```python
from build123d import *

# Parameters (mm, degrees)
SKETCH7_W           = 100
SKETCH7_H           = 14.5
BOSS_EXTRUDE1_DEPTH = 16.5
SKETCH8_R           = 5
CUT_EXTRUDE2_DEPTH  = 13
SKETCH10_R          = 13
CUT_EXTRUDE3_DEPTH  = 2
FILLET1_R           = 3
FILLET3_R           = 3
FILLET4_R           = 3
FILLET5_R           = 3


with BuildPart() as part:
    # Sketch7 → Boss-Extrude1 (new body)
    with BuildSketch(Plane(origin=(0, 0, 0), x_dir=(0, 1, 0), z_dir=(0, 0, 1))):
        Rectangle(SKETCH7_W, SKETCH7_H)
    extrude(amount=BOSS_EXTRUDE1_DEPTH)

    # Sketch8 → Cut-Extrude2 (cut)
    with BuildSketch(Plane(origin=(0, 0, 16.5), x_dir=(0, -1, 0), z_dir=(0, 0, 1))):
        with Locations(Location((0, 0, 0), (0, 0, 90))):
            Circle(SKETCH8_R)
    extrude(amount=-CUT_EXTRUDE2_DEPTH, mode=Mode.SUBTRACT)

    # Sketch10 → Cut-Extrude3 (cut)
    with BuildSketch(Plane.XY.offset(16.5)):
        with Locations((0, -31.55)):
            Circle(SKETCH10_R)
    cut_extrude3 = extrude(amount=-CUT_EXTRUDE3_DEPTH, mode=Mode.SUBTRACT)

    # Mirror1: Cut-Extrude3 across plane
    add(cut_extrude3.mirror(Plane.ZX), mode=Mode.SUBTRACT)

    # Fillet1
    fillet1_edges = [part.edges().sort_by_distance(p)[0] for p in [
        (-7.25, 0, 0),
    ]]
    fillet(fillet1_edges, radius=FILLET1_R)

    # Fillet3
    fillet3_edges = [part.edges().sort_by_distance(p)[0] for p in [
        (7.25, 0, 0),
    ]]
    fillet(fillet3_edges, radius=FILLET3_R)

    # Fillet4
    fillet4_edges = [part.edges().sort_by_distance(p)[0] for p in [
        (0, 50, 16.5),
    ]]
    fillet(fillet4_edges, radius=FILLET4_R)

    # Fillet5
    fillet5_edges = [part.edges().sort_by_distance(p)[0] for p in [
        (0, -50, 16.5),
    ]]
    fillet(fillet5_edges, radius=FILLET5_R)


solid = part.part
```
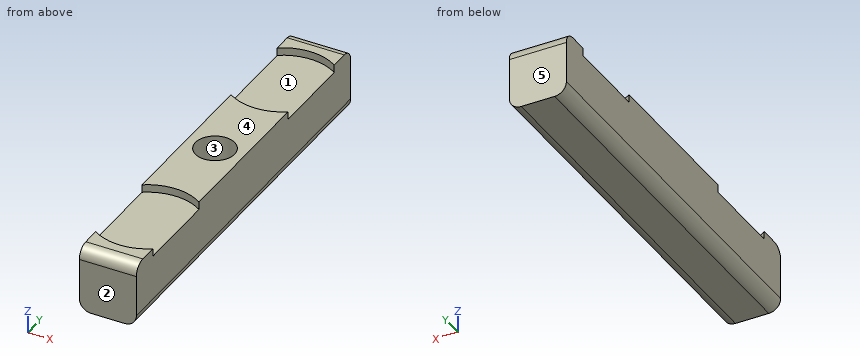
The model under review builds one solid part; all positions refer to its coordinate system, in mm. Face numbers are marked on the shaded views. A direction names the side the tool comes from. Give positions to 0.01 mm unless a question says otherwise; leave off trailing zeros. Write each loop counter-clockwise with the first axis right and the second up, starting at its lowest first coordinate (ties: lowest second). Pieces come first, ordered by that corner, then holes. Notation, with made-up numbers: M 23.5,50.25 L 76.5,50.25 A11 cw 76.5,56.25 Z; hole C 73,-23 d5. An arc over 180 degrees is marked long. Write each question's results on one line, items separated by ' | '. Start each with the question number.
1. Mouldability with a two-part tool opening along Y and no side actions: class the marked faces 3, 4 and 5 as released by +Y, released by -Y, zero draft, split by the parting line, or undercut.
2. We need section B-B (y = 0). Write out the cut boundary in (x, z).
3. For probe 1 along Y at (x, z) = (0, 13.25); probe 2 along Z at (x, y) = (3.75, 34); probe 3 along Y at (x, z) = (-1.25, 13.5), list the stretches that pass through material, from the lowest coordinate up. Write a range as [from, to].
4. Insertion check: pin 1 Ø4.5 at (x, y) = (1, 34.5) entering from +Z. The pin has a flat end and moves straight along its axis. Give the tip position at first contact, or say it passes through.
5. We need section D-D (y = -25.5). Write out the cut boundary in (x, z).
6. For the marked faces 1 and 2, list the 3-axis set-ups (+Z, -Z, +X, -X, +Y, -Y) from which the entire face can be reached by the end or side of a thin tool; tool diameter is ignored.
7. We need section A-A (z = 8.75). Write out the cut boundary in (x, y).
8. We need section C-C (x = -2.25). Write out the cut boundary in (y, z).
Results found:
1) face 3: undercut | face 4: zero draft | face 5: released by +Y
2) outline: M -7.25,3 A3 ccw -4.25,0 L 4.25,0 A3 ccw 7.25,3 L 7.25,16.5 L 5,16.5 L 5,3.5 L -5,3.5 L -5,16.5 L -7.25,16.5 Z
3) probe 1: y = [-50, -5], [5, 50] | probe 2: z = [0, 14.5] | probe 3: y = [-50, -4.84], [4.84, 50]
4) pin 1: stops at z = 14.5
5) outline: M -7.25,3 A3 ccw -4.25,0 L 4.25,0 A3 ccw 7.25,3 L 7.25,14.5 L -7.25,14.5 Z
6) face 1: +Z | face 2: +Z, -Z, +X, -X, -Y
7) outline: M -7.25,-50 L 7.25,-50 L 7.25,50 L -7.25,50 Z; hole C 0,0 d10
8) outline: M -50,0 L 50,0 L 50,13.5 A3 ccw 47,16.5 L 44.35,16.5 L 44.35,14.5 L 18.75,14.5 L 18.75,16.5 L 4.47,16.5 L 4.47,3.5 L -4.47,3.5 L -4.47,16.5 L -18.75,16.5 L -18.75,14.5 L -44.35,14.5 L -44.35,16.5 L -47,16.5 A3 ccw -50,13.5 Z
